Solid Edge part; units mm, degrees
sketch "Sketch1" plane through (0, 0, 0) normal (0, -1, 0) x (1, 0, 0)
  circle A0 centre (0, 0) radius 3.5
extrude "Protrusion1" add sketch "Sketch1" against normal blind 5
sketch "Sketch2" plane through (0, 5, 0) normal (0, 1, 0) x (-1, 0, 0)
  circle A0 centre (0, 0) radius 2.5
extrude "ExtrudedProtrusion_2" add sketch "Sketch2" along normal blind 16
fillet "Round_1" radius 0.2 1 edges at (-3.5, 0, 0)
sketch "Sketch3" plane through (0, 0, 0) normal (0, -1, 0) x (1, 0, 0)
  line L0 (0, 2.3094) -> (-2, 1.1547)
  line L1 (-2, 1.1547) -> (-2, -1.1547)
  line L2 (-2, -1.1547) -> (0, -2.3094)
  line L3 (0, -2.3094) -> (2, -1.1547)
  line L4 (2, -1.1547) -> (2, 1.1547)
  line L5 (2, 1.1547) -> (0, 2.3094)
extrude "ExtrudedCutout_2" cut sketch "Sketch3" against normal blind 2.3
properties material "Steel"
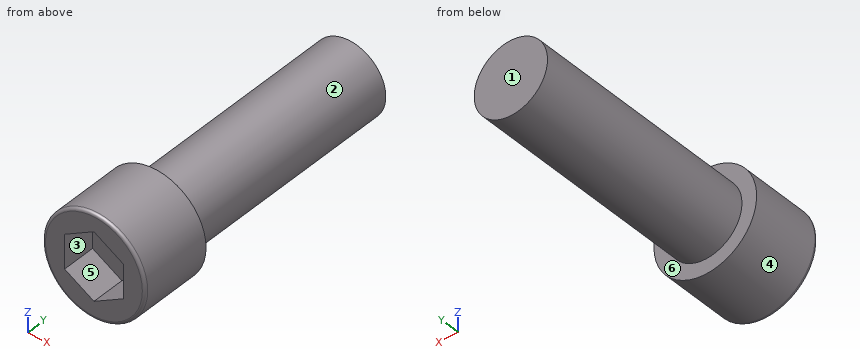
Work out the finished part from the listing and answer in its coordinate system (mm). Face numbers are marked on the shaded views. A direction names the side the tool comes from. Give positions to 0.01 mm unless a question says otherwise; leave off trailing zeros. Write each loop counter-clockwise with the first axis right and the second up, starting at its lowest first coordinate (ties: lowest second). Pieces come first, ordered by that corner, then holes. Notation, with made-up numbers: M -13,3.5 L 3,3.5 A12 cw 3,12.5 Z; hole C 67.5,24.5 d11. An arc over 180 degrees is marked long. Answer as CSV lines item,"result".
Q1. The mould has two halves that part along Z. Classify the marked faces 4, 5 and 6: +Z half, -Z half, draft (parallel to the pull), parting line (faces both ways), or undercut.
A:
face 4,"parting line"
face 5,"undercut"
face 6,"draft"
Q2. Given P1, Ø0.7, axis at y = 0.5, z = -0.5, coming from the +X side; P2, Ø1.2, axis at x = -0.5, z = 0.5, coming from the -Y side; P3, Ø4, axis at x = 2.5, y = 11, coming from the +Z side, each flat-ended and moving along its own axis, determine where each tip first touches the part or whether it passes through.
A:
P1,"stops at x = 3.5"
P2,"stops at y = 2.3"
P3,"stops at z = 2.45"
Q3. A cutting plane is placed at A-A on y = 2. Write down the section's boundary in (x, z).
A:
outline,"C 0,0 d7; hole M -2,-1.15 L 0,-2.31 L 2,-1.15 L 2,1.15 L 0,2.31 L -2,1.15 Z"
Q4. A cutting plane is placed at B-B on z = 0. Write down the section's boundary in (x, y).
A:
outline,"M -3.5,0.2 A0.2 ccw -3.3,0 L -2,0 L -2,2.3 L 2,2.3 L 2,0 L 3.3,0 A0.2 ccw 3.5,0.2 L 3.5,5 L 2.5,5 L 2.5,21 L -2.5,21 L -2.5,5 L -3.5,5 Z"
Q5. A tool of negligible diameter and unlimited length cuts with its end or side. For the marked faces 1, 2 and 3, from which of +Z, -Z, +X, -X, +Y, -Y can it reach the whole face along a straight path? Write none if from no direction.
A:
face 1,"+Z, -Z, +X, -X, +Y"
face 2,"+Y"
face 3,"-Y"
Q6. Find the intervals of material crossed by probe 1 along Y at (x, z) = (-1.75, -2.25); probe 2 along Y at (x, z) = (-0.5, 1.25); probe 3 along Z at (x, y) = (0, 6), in increasing order. Write a range as [from, to].
A:
probe 1,"y = [0, 5]"
probe 2,"y = [2.3, 21]"
probe 3,"z = [-2.5, 2.5]"
Q7. A cutting plane is placed at C-C on y = 11.25. Write down the section's boundary in (x, z).
A:
outline,"C 0,0 d5"
